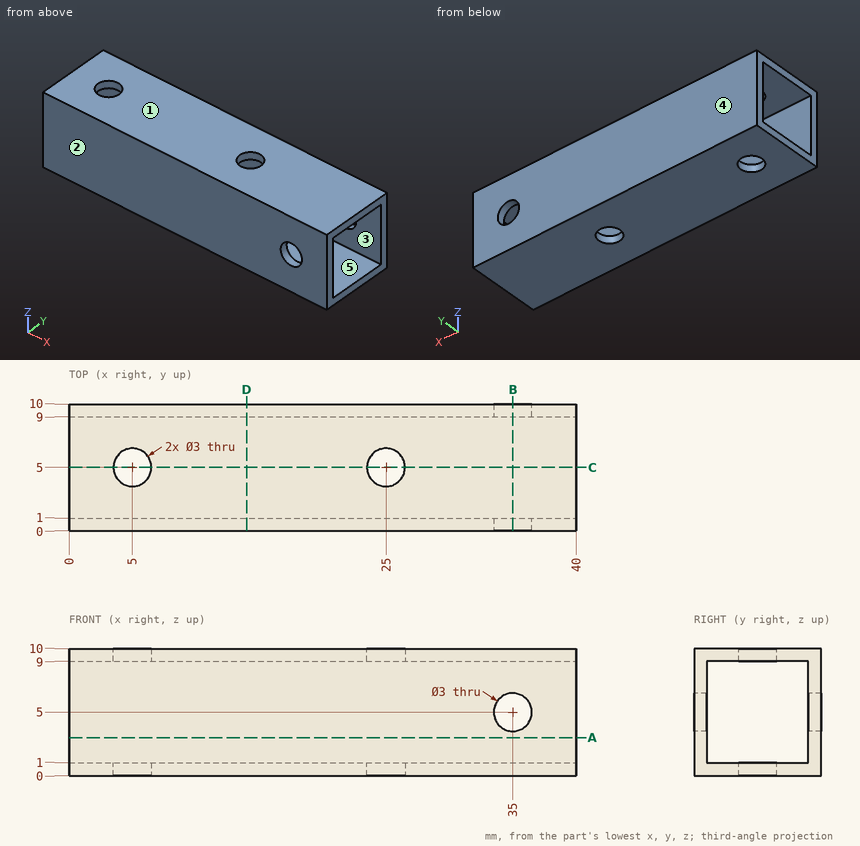
Geometry: see drawing. Coordinates: mm, zero at the bounding-box minimum. A direction names the side the tool comes from. Give positions to 0.01 mm unless a question says otherwise; leave off trailing zeros. Order: outer loops, then holes, each group sorted by start corner. A loop starts at its lowest first (then second) coordinate and runs counter-clockwise, first axis right, second up. Notation, with made-up numbers: (64, -36.75) - (80, -36.75) arc R24 ccw to (80, -24.75) - close; hole circle Ø1 at (86.25, 61.5). An arc over 180 degrees is marked (long way). Write each question's results on one line, items separated by ' | '.
Item 1: Section D-D (x = 14). Return loops of the section in (y, z).
A:
outline: (0, 0) - (10, 0) - (10, 10) - (0, 10) - close; hole (1, 1) - (9, 1) - (9, 9) - (1, 9) - close
Item 2: Section B-B (x = 35). Return loops of the section in (y, z).
A:
outline: (0, 0) - (10, 0) - (10, 3.5) - (9, 3.5) - (9, 1) - (1, 1) - (1, 3.5) - (0, 3.5) - close; (0, 6.5) - (1, 6.5) - (1, 9) - (9, 9) - (9, 6.5) - (10, 6.5) - (10, 10) - (0, 10) - close
Item 3: Section A-A (z = 3). Return loops of the section in (x, y).
A:
outline: (0, 0) - (40, 0) - (40, 1) - (0, 1) - close; (0, 9) - (40, 9) - (40, 10) - (0, 10) - close
Item 4: Material intervals for line 1 along Y through (x, z) = (19.5, 3.25); line 2 along Y through (x, z) = (25, 9.55), sorted ascending.
A:
line 1: y = 0 to 1, 9 to 10 | line 2: y = 0 to 3.5, 6.5 to 10
Item 5: Draft query along Z for the marked faces 1, 2 and 3. Return one class per face: released by +Z, released by -Z, zero draft, split by the parting line, or undercut.
A:
face 1: released by +Z | face 2: zero draft | face 3: undercut
Item 6: Access query for the marked faces 4 and 5. Directions: +Z, -Z, +X, -X, +Y, -Y. A direction counts if a zero-diameter tool reaches every point of the face in a straight line with its end or side. Return the directions, or none.
A:
face 4: +Z, -Z, +X, -X, +Y | face 5: +X, -X
Item 7: Section C-C (y = 5). Return loops of the section in (x, z).
A:
outline: (0, 0) - (3.5, 0) - (3.5, 1) - (0, 1) - close; (0, 9) - (3.5, 9) - (3.5, 10) - (0, 10) - close; (6.5, 0) - (23.5, 0) - (23.5, 1) - (6.5, 1) - close; (6.5, 9) - (23.5, 9) - (23.5, 10) - (6.5, 10) - close; (26.5, 0) - (40, 0) - (40, 1) - (26.5, 1) - close; (26.5, 9) - (40, 9) - (40, 10) - (26.5, 10) - close
